Check sheet for the modelled part. Datum: model origin and axes. Units: mm. A direction names the side the tool comes from. Round coordinates to 2 decimals unless told otherwise and drop trailing zeros. Write each loop counter-clockwise with the first axis right and the second up, starting at its lowest first coordinate (ties: lowest second). Pieces come first, ordered by that corner, then holes. Notation, with made-up numbers: (-12, 5) -> (41, 5) arc R27 ccw to (41, 42) -> close; hole circle Ø1 at (71, -17). An arc over 180 degrees is marked (long way). One line per item, written item: value.
from build123d import *

# Parameters (mm, degrees)
SKETCH1_W            = 25
SKETCH1_H            = 23.862
PCB_BOARD_DEPTH      = 1
PCB_CORNER_FILLETS_R = 2
SKETCH2_R            = 1.1
MOUNTING_HOLES_DEPTH = 18.308921428
SKETCH3_W            = 8.5
SKETCH3_H            = 8.5
SENSOR_HOUSING_DEPTH = 3.5
SKETCH4_R            = 3.6
LENS_BARREL_DEPTH    = 1.4
SKETCH5_R            = 1.8
LENS_APERTURE_DEPTH  = 0.8
SKETCH6_W            = 21
SKETCH6_H            = 5.5
CSI_CONNECTOR_DEPTH  = 2.5
SKETCH7_W            = 9
SKETCH7_H            = 4
FLEX_CONNECTOR_DEPTH = 1.5


with BuildPart() as part:
    # Sketch1 → PCB_Board (new body)
    with BuildSketch(Plane.XY):
        Rectangle(SKETCH1_W, SKETCH1_H)
    extrude(amount=PCB_BOARD_DEPTH)

    # PCB_Corner_Fillets
    pcb_corner_fillets_edges = [part.edges().sort_by_distance(p)[0] for p in [
        (-12.5, 11.931, 0.5),
        (12.5, 11.931, 0.5),
        (12.5, -11.931, 0.5),
        (-12.5, -11.931, 0.5),
    ]]
    fillet(pcb_corner_fillets_edges, radius=PCB_CORNER_FILLETS_R)

    # Sketch2 → Mounting_Holes (cut, through all)
    with BuildSketch(Plane.XY.offset(1)):
        with Locations((10.5, 9.931)):
            Circle(SKETCH2_R)
        with Locations((-10.5, 9.931)):
            Circle(SKETCH2_R)
        with Locations((10.5, -2.569)):
            Circle(SKETCH2_R)
        with Locations((-10.5, -2.569)):
            Circle(SKETCH2_R)
    extrude(amount=-MOUNTING_HOLES_DEPTH, mode=Mode.SUBTRACT)

    # Sketch3 → Sensor_Housing (add)
    with BuildSketch(Plane.XY.offset(1)):
        with Locations((0, 2.469)):
            Rectangle(SKETCH3_W, SKETCH3_H)
    extrude(amount=SENSOR_HOUSING_DEPTH)

    # Sketch4 → Lens_Barrel (add)
    with BuildSketch(Plane.XY.offset(4.5)):
        with Locations((0, 2.469)):
            Circle(SKETCH4_R)
    extrude(amount=LENS_BARREL_DEPTH)

    # Sketch5 → Lens_Aperture (cut)
    with BuildSketch(Plane.XY.offset(5.9)):
        with Locations((0, 2.469)):
            Circle(SKETCH5_R)
    extrude(amount=-LENS_APERTURE_DEPTH, mode=Mode.SUBTRACT)

    # Sketch6 → CSI_Connector (add)
    with BuildSketch(Plane(origin=(0, 0, 0), x_dir=(-1, 0, 0), z_dir=(0, 0, -1))):
        with Locations((0, -9.181)):
            Rectangle(SKETCH6_W, SKETCH6_H)
    extrude(amount=CSI_CONNECTOR_DEPTH)

    # Sketch7 → Flex_Connector (add)
    with BuildSketch(Plane.XY.offset(1)):
        with Locations((0, -5.8)):
            Rectangle(SKETCH7_W, SKETCH7_H)
    extrude(amount=FLEX_CONNECTOR_DEPTH)


solid = part.part
Item 1: Mould release check, pull along Y, two halves, no side actions. Record for faces 1 (the cylindrical face through (-9.45, -2.24, 0.51)), 2 (the flat face through (12.5, -0.1, 0.5)), 3 (the cylindrical face through (-0.47, 6.04, 5.19)): pulls with the +Y half, pulls with the -Y half, needs draft (parallel to the pull), parting line crosses it, or undercut.
Answer:
face 1: undercut
face 2: needs draft
face 3: parting line crosses it
Item 2: Thickness scan on line 1 (Y direction, x = 10.5, z = 0.85); line 2 (Y direction, x = 0, z = 5.6); line 3 (Y direction, x = -2.5, z = 1.75). Record the ranges inside material, lowest first.
Answer:
line 1: y = -11.93 to -3.67, -1.47 to 8.83, 11.03 to 11.93
line 2: y = -1.13 to 0.67, 4.27 to 6.07
line 3: y = -7.8 to -3.8, -1.78 to 6.72
Item 3: Sectioned sample at A-A on x = 0. Enter the section's corners in (y, z), and give its area (3 significant figures).
Answer:
outline: (-11.93, -2.5) -> (-6.43, -2.5) -> (-6.43, 0) -> (11.93, 0) -> (11.93, 1) -> (6.72, 1) -> (6.72, 4.5) -> (6.07, 4.5) -> (6.07, 5.9) -> (4.27, 5.9) -> (4.27, 5.1) -> (0.67, 5.1) -> (0.67, 5.9) -> (-1.13, 5.9) -> (-1.13, 4.5) -> (-1.78, 4.5) -> (-1.78, 1) -> (-3.8, 1) -> (-3.8, 2.5) -> (-7.8, 2.5) -> (-7.8, 1) -> (-11.93, 1) -> close
area: 80.6 mm^2
Item 4: Sectioned sample at B-B on y = 10.5. Enter the section's corners in (x, z).
Answer:
outline: (-12.42, 0) -> (-11.44, 0) -> (-11.44, 1) -> (-12.42, 1) -> close; (-9.56, 0) -> (9.56, 0) -> (9.56, 1) -> (-9.56, 1) -> close; (11.44, 0) -> (12.42, 0) -> (12.42, 1) -> (11.44, 1) -> close
Item 5: Depth check by flat-ended pin: P1, Ø1.5, axis at y = 7, z = 4, coming from the -X side; P2, Ø1.5, axis at x = 4, z = -0.5, coming from the +Y side; P3, Ø5, axis at x = -6, y = 7, coming from the -Z side; P4, Ø1, axis at y = 2, z = 2.5, coming from the +X side. Enter the tip coordinate at first touch or a pass-through.
Answer:
P1: stops at x = -4.25
P2: stops at y = 11.93
P3: stops at z = 0
P4: stops at x = 4.25
Item 6: Sectioned sample at C-C on z = 3.5. Enter the section's corners in (x, y).
Answer:
outline: (-4.25, -1.78) -> (4.25, -1.78) -> (4.25, 6.72) -> (-4.25, 6.72) -> close
Item 7: Sectioned sample at D-D on y = -0.5. Enter the section's corners in (x, z), and give its area (3 significant figures).
Answer:
outline: (-12.5, 0) -> (12.5, 0) -> (12.5, 1) -> (4.25, 1) -> (4.25, 4.5) -> (2.04, 4.5) -> (2.04, 5.9) -> (-2.04, 5.9) -> (-2.04, 4.5) -> (-4.25, 4.5) -> (-4.25, 1) -> (-12.5, 1) -> close
area: 60.5 mm^2
Item 8: Tool access check on faces 4 (the flat face through (4.5, -6, 2)), 5 (the flat face through (0, 6.719, 3)), 6 (the flat face through (0, -1.781, 3)). Record the directions out of +Z, -Z, +X, -X, +Y, -Y that give a thin tool (end or side, any length) a straight path to the whole face; none if there is none.
Answer:
face 4: +Z, +X, +Y, -Y
face 5: +Z, +X, -X, +Y
face 6: +Z, +X, -X
